CAD build for the part. Positions are in the model's coordinates, mm. Face numbers are marked on the shaded views. A direction names the side the tool comes from. Round coordinates to 2 decimals unless told otherwise and drop trailing zeros. Loops run counter-clockwise (first coordinate to the right, second up) from the corner with the lowest first, then second, coordinate; pieces in that order, holes last. Notation, with made-up numbers: M -5.5,-13.75 L 31.5,-13.75 A22 ccw 31.5,5.25 Z; hole C 41.5,47.25 d2. An arc over 180 degrees is marked long. Use a Markdown table: item, result. Add a question column.
(1) Flat gauge pins, fed straight in: P1, Ø12, axis at y = -15, z = 23.5, coming from the +X side; P2, Ø2.5, axis at x = 11.57, y = 7.51, coming from the +Z side; P3, Ø3.5, axis at y = 7.5, z = -2, coming from the -X side; P4, Ø5, axis at x = -14.16, y = 7.51, coming from the +Z side. Where does each tip first touch, or does it go through?
(2) Which spindle directions (+Z, -Z, +X, -X, +Y, -Y) get a long thin tool onto all of the face, cutting with end or side? Do the marked faces 5 and 6. Say none if no direction does.
(3) Wall check: L1, parallel to X at y = -7, z = 3.5; L2, parallel to Z at x = -4, y = 5.5; L3, parallel to Z at x = -22, y = 6.5. Give the ranges that are in metal, low to high.
(4) Band-saw the part on C-C, the plane y = -10. Write the cut outline in (x, z).
(5) Band-saw the part on A-A, the plane y = 4.5. Write the cut outline in (x, z), and give its area (3 significant figures).
(6) Band-saw the part on B-B, the plane z = 16. Write the cut outline in (x, y), and give its area (3 significant figures).
(7) Two-plate mould, pull along X, no slides. Class the marked faces 1, 2, 3 and 4: released by +X, released by -X, zero draft, split by the parting line, or undercut.
(8) Band-saw the part on D-D, the plane x = 16.5. Write the cut outline in (y, z), and give its area (3 significant figures).
from build123d import *

# Parameters (mm, degrees)
ESBO_O1_W                        = 48
ESBO_O1_H                        = 39
FLANGE_BASE1_DEPTH               = 3
ESBO_O6_R                        = 2.3
CORTE_EXTRUS_O1_DEPTH            = 10
ARESTA_FLANGE1_STRIP_W           = 13.4732
ARESTA_FLANGE1_STRIP_H           = 3
ARESTA_FLANGE1_STRIP_CUT_DEPTH   = 39
ARESTA_FLANGE1_STRIP_2_W         = 13.4732
ARESTA_FLANGE1_STRIP_2_H         = 3
ARESTA_FLANGE1_STRIP_CUT_2_DEPTH = 39
ARESTA_FLANGE1_DEPTH             = 39
ARESTA_FLANGE1_BEND_DEPTH        = 39
ESBO_O13_R                       = 2.3
CORTE_EXTRUS_O2_DEPTH            = 70
FILETE1_R                        = 5
ESBO_O14_R                       = 1.997873176
ESBO_O14_R_2                     = 2.026064888
ESBO_O14_R_3                     = 2
CORTE_EXTRUS_O4_DEPTH            = 3


# Sheet-metal steps are written as plain solids
with BuildPart() as part:
    # Esboço1 → Flange-base1 (new body)
    with BuildSketch(Plane.XY):
        with Locations((2.993735783, -4.490936556)):
            Rectangle(ESBO_O1_W, ESBO_O1_H)
    extrude(amount=-FLANGE_BASE1_DEPTH)

    # Esboço6 → Corte-extrusão1 (cut)
    with BuildSketch(Plane.XY):
        with BuildLine():
            Line((-14.156264217, 5.509063444), (-14.156264217, 7.509063444))
            Line((-14.156264217, 7.509063444), (-12.156264217, 7.509063444))
            ThreePointArc((-12.156264217, 7.509063444), (-15.570477779, 8.923277006), (-14.156264217, 5.509063444))
        make_face()
        with BuildLine():
            Line((-12.156264217, 7.509063444), (-14.156264217, 7.509063444))
            Line((-14.156264217, 7.509063444), (-14.156264217, 5.509063444))
            ThreePointArc((-14.156264217, 5.509063444), (-12.742050654, 6.094849882), (-12.156264217, 7.509063444))
        make_face()
        with BuildLine():
            ThreePointArc((-12.156264217, -16.490936556), (-12.742050654, -15.076722994), (-14.156264217, -14.490936556))
            Line((-14.156264217, -14.490936556), (-14.156264217, -16.490936556))
            Line((-14.156264217, -16.490936556), (-12.156264217, -16.490936556))
        make_face()
        with BuildLine():
            Line((-14.156264217, -16.490936556), (-14.156264217, -14.490936556))
            ThreePointArc((-14.156264217, -14.490936556), (-15.570477779, -17.905150118), (-12.156264217, -16.490936556))
            Line((-12.156264217, -16.490936556), (-14.156264217, -16.490936556))
        make_face()
        with Locations((2.993735783, -4.490936556)):
            Circle(ESBO_O6_R)
        with BuildLine():
            Line((4.493735783, 7.509063444), (1.493735783, 7.509063444))
            Line((1.493735783, 7.509063444), (1.493735783, 3.523823043))
            ThreePointArc((1.493735783, 3.523823043), (2.993735783, 2.023823043), (4.493735783, 3.523823043))
            Line((4.493735783, 3.523823043), (4.493735783, 7.509063444))
        make_face()
        with BuildLine():
            Line((1.493735783, 12.523823043), (1.493735783, 7.509063444))
            Line((1.493735783, 7.509063444), (4.493735783, 7.509063444))
            Line((4.493735783, 7.509063444), (4.493735783, 12.523823043))
            ThreePointArc((4.493735783, 12.523823043), (2.993735783, 14.023823043), (1.493735783, 12.523823043))
        make_face()
        with BuildLine():
            Line((1.493735783, -12.505696155), (1.493735783, -16.490936556))
            Line((1.493735783, -16.490936556), (4.493735783, -16.490936556))
            Line((4.493735783, -16.490936556), (4.493735783, -12.505696155))
            ThreePointArc((4.493735783, -12.505696155), (2.993735783, -11.005696155), (1.493735783, -12.505696155))
        make_face()
        with BuildLine():
            Line((4.493735783, -16.490936556), (1.493735783, -16.490936556))
            Line((1.493735783, -16.490936556), (1.493735783, -21.505696155))
            ThreePointArc((1.493735783, -21.505696155), (2.993735783, -23.005696155), (4.493735783, -21.505696155))
            Line((4.493735783, -21.505696155), (4.493735783, -16.490936556))
        make_face()
        with BuildLine():
            ThreePointArc((22.143735783, -16.490936556), (21.557949346, -15.076722994), (20.143735783, -14.490936556))
            Line((20.143735783, -14.490936556), (20.143735783, -16.490936556))
            Line((20.143735783, -16.490936556), (18.143735783, -16.490936556))
            ThreePointArc((18.143735783, -16.490936556), (20.143735783, -18.490936556), (22.143735783, -16.490936556))
        make_face()
        with BuildLine():
            Line((20.143735783, -16.490936556), (20.143735783, -14.490936556))
            ThreePointArc((20.143735783, -14.490936556), (18.729522221, -15.076722994), (18.143735783, -16.490936556))
            Line((18.143735783, -16.490936556), (20.143735783, -16.490936556))
        make_face()
        with BuildLine():
            ThreePointArc((22.143735783, 7.509063444), (20.143735783, 9.509063444), (18.143735783, 7.509063444))
            Line((18.143735783, 7.509063444), (20.143735783, 7.509063444))
            Line((20.143735783, 7.509063444), (20.143735783, 5.509063444))
            ThreePointArc((20.143735783, 5.509063444), (21.557949346, 6.094849882), (22.143735783, 7.509063444))
        make_face()
        with BuildLine():
            Line((20.143735783, 7.509063444), (18.143735783, 7.509063444))
            ThreePointArc((18.143735783, 7.509063444), (18.729522221, 6.094849882), (20.143735783, 5.509063444))
            Line((20.143735783, 5.509063444), (20.143735783, 7.509063444))
        make_face()
    extrude(amount=-CORTE_EXTRUS_O1_DEPTH, mode=Mode.SUBTRACT)

    # Aresta-Flange1 strip (across the edge) → Aresta-Flange1 strip cut (cut)
    with BuildSketch(Plane(origin=(26.993735783, -23.990936556, 0), x_dir=(-1, 0, 0), z_dir=(0, 1, 0))):
        with Locations((-6, -1.5)):
            Rectangle(ARESTA_FLANGE1_STRIP_W, ARESTA_FLANGE1_STRIP_H)
    extrude(amount=ARESTA_FLANGE1_STRIP_CUT_DEPTH, mode=Mode.SUBTRACT)

    # Aresta-Flange1 strip 2 (across the edge) → Aresta-Flange1 strip cut 2 (cut)
    with BuildSketch(Plane(origin=(-21.006264217, 15.009063444, 0), x_dir=(1, 0, 0), z_dir=(0, -1, 0))):
        with Locations((-6, -1.5)):
            Rectangle(ARESTA_FLANGE1_STRIP_2_W, ARESTA_FLANGE1_STRIP_2_H)
    extrude(amount=ARESTA_FLANGE1_STRIP_CUT_2_DEPTH, mode=Mode.SUBTRACT)

    # Aresta-Flange1 section (across the edge) → Aresta-Flange1 (add)
    with BuildSketch(Plane(origin=(26.993735783, -23.990936556, 0), x_dir=(-1, 0, 0), z_dir=(0, 1, 0))):
        with BuildLine():
            Line((-3, 0.7366), (-3, 30))
            Line((-3, 30), (0, 30))
            Line((0, 30), (0, 0.7366))
            ThreePointArc((0, 0.7366), (0.215745145, 0.215745145), (0.7366, 0))
            Line((0.7366, 0), (0.7366, -3))
            ThreePointArc((0.7366, -3), (-1.905575199, -1.905575199), (-3, 0.7366))
        make_face()
    extrude(amount=ARESTA_FLANGE1_DEPTH)

    # Aresta-Flange1 section 2 (across the edge) → Aresta-Flange1 bend (add)
    with BuildSketch(Plane(origin=(-21.006264217, 15.009063444, 0), x_dir=(1, 0, 0), z_dir=(0, -1, 0))):
        with BuildLine():
            Line((-3, 0.7366), (-3, 30))
            Line((-3, 30), (0, 30))
            Line((0, 30), (0, 0.7366))
            ThreePointArc((0, 0.7366), (0.215745145, 0.215745145), (0.7366, 0))
            Line((0.7366, 0), (0.7366, -3))
            ThreePointArc((0.7366, -3), (-1.905575199, -1.905575199), (-3, 0.7366))
        make_face()
    extrude(amount=ARESTA_FLANGE1_BEND_DEPTH)

    # Esboço13 → Corte-extrusão2 (cut)
    with BuildSketch(Plane.ZY.offset(24.006264217)):
        with Locations((26.166238029, -6.281221748)):
            Circle(ESBO_O13_R)
        Polygon((0.7366, -23.990936556), (30, -23.990936556), (30, -9.490936556), align=None)
        with BuildLine():
            ThreePointArc((26.391219924, 3.216113833), (19.60969386, 0.593494869), (16.668902447, -6.056239853))
            ThreePointArc((16.668902447, -6.056239853), (18.620976907, -8.103043532), (20.667780587, -6.150969072))
            ThreePointArc((20.667780587, -6.150969072), (22.370344036, -2.301122654), (26.296490705, -0.782764306))
            ThreePointArc((26.296490705, -0.782764306), (28.343294384, 1.169310154), (26.391219924, 3.216113833))
        make_face()
    extrude(amount=-CORTE_EXTRUS_O2_DEPTH, mode=Mode.SUBTRACT)

    # Filete1
    filete1_edges = [part.edges().sort_by_distance(p)[0] for p in [
        (28.493735783, 15.009063444, 30),
        (-22.506264217, 15.009063444, 30),
        (-22.506264217, -9.490936556, 30),
        (28.493735783, -9.490936556, 30),
    ]]
    fillet(filete1_edges, radius=FILETE1_R)

    # Esboço14 → Corte-extrusão4 (cut)
    with BuildSketch(Plane.XY):
        with Locations((-5.581264217, 7.509063444)):
            Circle(ESBO_O14_R)
        with Locations((11.568735783, 7.509063444)):
            Circle(ESBO_O14_R_2)
        with Locations((13.493735783, -2.990936556)):
            Circle(ESBO_O14_R_3)
        with Locations(Location((-7.506264217, -2.990936556, 0), (0, 0, 180))):
            Circle(ESBO_O14_R_3)
    extrude(amount=-CORTE_EXTRUS_O4_DEPTH, mode=Mode.SUBTRACT)


solid = part.part
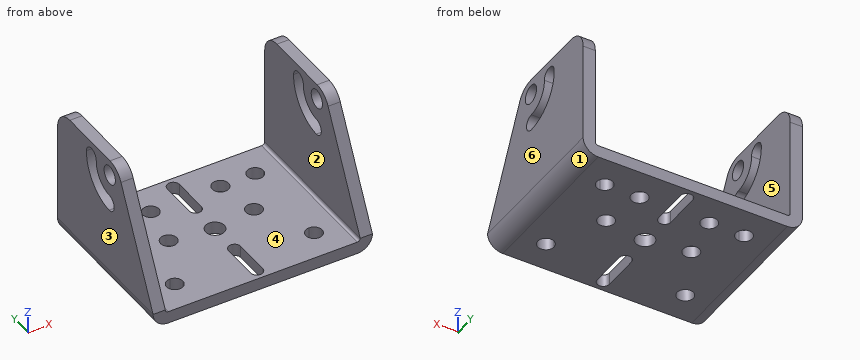
Return value:
| question | item | result |
|---|---|---|
| 1 | P1 | x = 29.99 |
| 1 | P2 | through |
| 1 | P3 | x = -23.87 |
| 1 | P4 | z = 0 |
| 2 | face 5 | +Z, +Y, -Y |
| 2 | face 6 | +Z, -Z, +X, +Y, -Y |
| 3 | L1 | -24.01 to -21.01, 26.99 to 29.99 |
| 3 | L2 | -3 to 0 |
| 3 | L3 | -2.58 to 30 |
| 4 | outline | M -24.01,0.74 A3.74 ccw -20.27,-3 L 26.26,-3 A3.74 ccw 29.99,0.74 L 29.99,28.46 L 26.99,28.46 L 26.99,0.74 A0.74 cw 26.26,0 L -20.27,0 A0.74 cw -21.01,0.74 L -21.01,28.46 L -24.01,28.46 Z |
| 5 | outline | M -24.01,0.74 A3.74 ccw -20.27,-3 L 1.49,-3 L 1.49,0 L -20.27,0 A0.74 cw -21.01,0.74 L -21.01,30 L -24.01,30 Z; M 4.49,-3 L 26.26,-3 A3.74 ccw 29.99,0.74 L 29.99,30 L 26.99,30 L 26.99,0.74 A0.74 cw 26.26,0 L 4.49,0 Z |
| 5 | area | 327 mm^2 |
| 6 | outline | M -24.01,-16.43 L -21.01,-16.43 L -21.01,15.01 L -24.01,15.01 Z; M 26.99,-16.43 L 29.99,-16.43 L 29.99,15.01 L 26.99,15.01 Z |
| 6 | area | 189 mm^2 |
| 7 | face 1 | released by +X |
| 7 | face 2 | undercut |
| 7 | face 3 | released by -X |
| 7 | face 4 | undercut |
| 8 | outline | M -23.99,-3 L 15.01,-3 L 15.01,0 L -23.99,0 Z |
| 8 | area | 117 mm^2 |
